from build123d import *

# Parameters (mm, degrees)
ESQUISSE1_R             = 2.5
BASE_EXTRUSION_DEPTH    = 1.5
ESQUISSE2_R             = 1.5
BOSS_EXTRU_1_DEPTH      = 23
CHANFREIN1_SIZE         = 0.25
ESQUISSE3_W             = 1
ESQUISSE3_H             = 8
ENL_V_MAT_EXTRU_1_DEPTH = 0.75
CONG_1_R                = 0.5


with BuildPart() as part:
    # Esquisse1 → Base-Extrusion (new body)
    with BuildSketch(Plane.XY):
        Circle(ESQUISSE1_R)
    extrude(amount=BASE_EXTRUSION_DEPTH)

    # Esquisse2 → Boss.-Extru.1 (add)
    with BuildSketch(Plane.XY.offset(1.5)):
        Circle(ESQUISSE2_R)
    extrude(amount=BOSS_EXTRU_1_DEPTH)

    # Chanfrein1
    chanfrein1_edges = [part.edges().sort_by_distance(p)[0] for p in [
        (-1.5, 0, 24.5),
    ]]
    chamfer(chanfrein1_edges, length=CHANFREIN1_SIZE)

    # Esquisse3 → Enlèv. mat.-Extru.1 (cut)
    with BuildSketch(Plane(origin=(0, 0, 0), x_dir=(-1, 0, 0), z_dir=(0, 0, -1))):
        with Locations((0, -1)):
            Rectangle(ESQUISSE3_W, ESQUISSE3_H)
    extrude(amount=-ENL_V_MAT_EXTRU_1_DEPTH, mode=Mode.SUBTRACT)

    # Congé1
    cong_1_edges = [part.edges().sort_by_distance(p)[0] for p in [
        (1.936491673, 1.58113883, 0),
        (-2.5, 0, 0),
        (1.936491673, -1.58113883, 0),
    ]]
    fillet(cong_1_edges, radius=CONG_1_R)


solid = part.part
CAD build for the part. Positions are in the model's coordinates, mm. A direction names the side the tool comes from. Round coordinates to 2 decimals unless told otherwise and drop trailing zeros. Write each loop counter-clockwise with the first axis right and the second up, starting at its lowest first coordinate (ties: lowest second). Pieces come first, ordered by that corner, then holes. Notation, with made-up numbers: M 31.25,20.25 L 43.25,20.25 A22 ccw 43.25,53.25 Z; hole C 28.25,61.25 d4. An arc over 180 degrees is marked long. Put each result on its own line as item: value. Start each with the question number.
1) Pin check, flat tips, straight feed: pin 1 Ø1 at (x, y) = (1.5, 1) entering from -Z; pin 2 Ø0.5 at (x, y) = (0, 1) entering from -Z; pin 3 Ø1 at (x, z) = (-1.5, 4) entering from -Y. Stop position of each tip, or through.
2) Saw through at C-C, the plane z = 6.5. Write the cut outline in (x, y), and give its area (3 significant figures).
3) 3-axis set-ups, long thin cutter, end or side, ignore diameter. For faces 1 (the flat face through (0, 0, 0.75)), 2 (the cylindrical face through (-0.54, -2.44, 0.99)), 3 (the flat face through (0, -2, 1.5)): which of +Z, -Z, +X, -X, +Y, -Y reach the whole face in a straight line?
4) Saw through at A-A, the plane x = 0. Write the cut outline in (y, z), and give its area (3 significant figures).
5) Saw through at B-B, the plane y = 0. Write the cut outline in (x, z), and give its area (3 significant figures).
6) Drill centre lines: probe 1 along Z at (x, y) = (1.65, -0.6); probe 2 along Z at (x, y) = (0.35, -1.85); probe 3 along X at (y, z) = (1.3, 3.5). Where is each one in solid material? Low to high. Write a range as [from, to].
Resolved:
1. pin 1: z = 0
1. pin 2: z = 0.75
1. pin 3: y = -1.12
2. outline: C 0,0 d3
2. area: 7.07 mm²
3. face 1: -Z, +Y, -Y
3. face 2: +Z, -Z
3. face 3: +Z
4. outline: M -2.5,0.75 L 2.5,0.75 L 2.5,1.5 L 1.5,1.5 L 1.5,24.25 L 1.25,24.5 L -1.25,24.5 L -1.5,24.25 L -1.5,1.5 L -2.5,1.5 Z
4. area: 72.7 mm²
5. outline: M -2.5,0.5 A0.5 ccw -2,0 L -0.5,0 L -0.5,0.75 L 0.5,0.75 L 0.5,0 L 2,0 A0.5 ccw 2.5,0.5 L 2.5,1.5 L 1.5,1.5 L 1.5,24.25 L 1.25,24.5 L -1.25,24.5 L -1.5,24.25 L -1.5,1.5 L -2.5,1.5 Z
5. area: 75.6 mm²
6. probe 1: [0, 1.5]
6. probe 2: [0.75, 1.5]
6. probe 3: [-0.75, 0.75]
